The drawing under review shows one solid part. Ordinate dimensions are in mm from its lowest x, y, z. A direction names the side the tool comes from. Round coordinates to 2 decimals unless told otherwise and drop trailing zeros. Write each loop counter-clockwise with the first axis right and the second up, starting at its lowest first coordinate (ties: lowest second). Pieces come first, ordered by that corner, then holes. Notation, with made-up numbers: (44, -15.75) - (84, -15.75) arc R22 cw to (84, 21.25) - close; hole circle Ø10 at (-10, -31.75). An arc over 180 degrees is marked (long way). One line per question, with ' | ' between items. Start each with the question number.
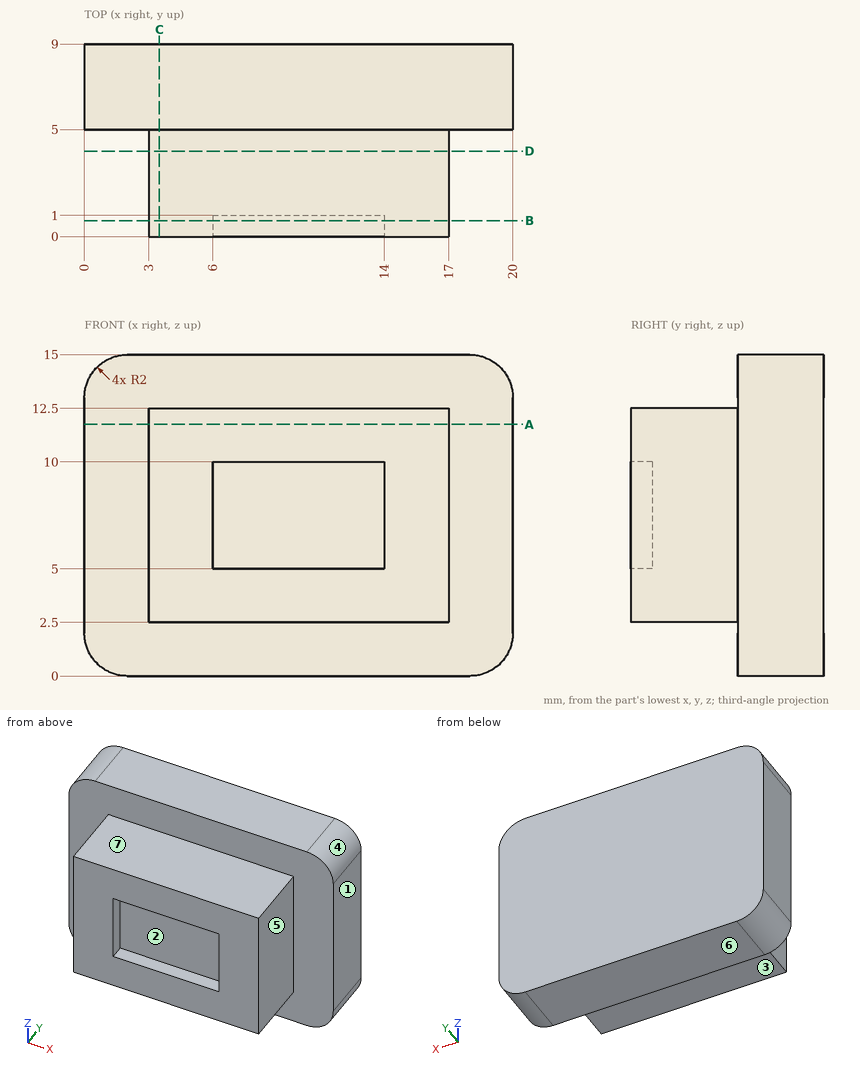
1. Add section C-C, the plane x = 3.5. Write out the cut boundary in (y, z).
2. The part is to be moulded in two halves that separate along Z. For the marked faces 1, 2, 3 and 4, say which applies: pulls with the +Z half, pulls with the -Z half, needs draft (parallel to the pull), parting line crosses it, or undercut.
3. Add section B-B, the plane y = 0.75. Write out the cut boundary in (x, z).
4. Machinability: for the marked faces 5, 6 and 7, which of the approach directions +Z, -Z, +X, -X, +Y, -Y give a long, thin tool a straight path to every point of the face, cutting with its end or side? Answer none if there is none.
5. Wall thickness on line 1 along Y through (x, z) = (11.25, 6.5); line 2 along X through (y, z) = (4.5, 10.25); line 3 along Z through (x, y) = (14.75, 1): over which ranges is each line inside the solid? List them lowest first. Write a range as [from, to].
6. Add section A-A, the plane z = 11.75. Write out the cut boundary in (x, y).
7. Clearance check with flat-ended pins moving along their axes: P1, Ø5, axis at y = 1.5, z = 5.5, coming from the -X side; P2, Ø2.5, axis at x = 13.5, y = 3.5, coming from the -Z side; P3, Ø1, axis at y = 1.5, z = 4.5, coming from the +X side. State where each tip first meets the part, or that it passes through.
8. Add section D-D, the plane y = 4. Write out the cut boundary in (x, z), then the cut area to 3 significant figures.
Geometry check:
1) outline: (0, 2.5) - (5, 2.5) - (5, 0) - (9, 0) - (9, 15) - (5, 15) - (5, 12.5) - (0, 12.5) - close
2) face 1: needs draft | face 2: undercut | face 3: pulls with the -Z half | face 4: pulls with the +Z half
3) outline: (3, 2.5) - (17, 2.5) - (17, 12.5) - (3, 12.5) - close; hole (6, 5) - (14, 5) - (14, 10) - (6, 10) - close
4) face 5: +Z, -Z, +X, -Y | face 6: -Z, +X, -X, +Y, -Y | face 7: +Z, +X, -X, -Y
5) line 1: y = [1, 9] | line 2: x = [3, 17] | line 3: z = [2.5, 12.5]
6) outline: (0, 5) - (3, 5) - (3, 0) - (17, 0) - (17, 5) - (20, 5) - (20, 9) - (0, 9) - close
7) P1: stops at x = 3 | P2: stops at z = 2.5 | P3: stops at x = 17
8) outline: (3, 2.5) - (17, 2.5) - (17, 12.5) - (3, 12.5) - close | area: 140 mm2
